Input: part model. Units: mm. Frame: model coordinates. A direction names the side the tool comes from. Coordinates: 2 decimals unless noted, no trailing zeros. Order: outer loops, then holes, each group sorted by start corner. A loop starts at its lowest first (then second) coordinate and runs counter-clockwise, first axis right, second up. Notation, with made-up numbers: M -8,49.25 L 17,49.25 A34 ccw 17,85.25 Z; hole C 67,75.25 d6. An arc over 180 degrees is marked long. Answer in a Markdown table with one row per item.
Autodesk Inventor part; units mm, degrees
ref_plane "Work Plane1" through (0, 10, 0) normal (0, 1, 0) x (-1, 0, 0)
ref_plane "YZ Plane" through (0, 0, 0) normal (1, 0, 0) x (0, 1, 0)
ref_plane "XY Plane" through (0, 0, 0) normal (0, 0, 1) x (1, 0, 0)
sketch "Sketch1" plane through (0, 0, 0) normal (0, 0, 1) x (1, 0, 0)
  line L0 (-50, 0) -> (0, 0)
  line L1 (0, 0) -> (50, 0)
  line L2 (-50, 0) -> (-50, 6)
  line L3 (-50, 6) -> (-33, 6)
  line L4 (-33, 6) -> (-33, 10)
  line L5 (-33, 10) -> (33, 10)
  line L6 (33, 10) -> (33, 6)
  line L7 (33, 6) -> (50, 6)
  line L8 (50, 6) -> (50, 0)
  point P0 (-33, 8)
  dimension "d0" = 100
  dimension "d1" = 12
  dimension "d2" = 20
  dimension "d3" = 17
  dimension "d4" = 83
revolve "Revolution1" add sketch "Sketch1" angle 360 about axis through (-50, 0, 0) along (1, 0, 0)
sketch "Sketch2" plane through (-50, 0, 0) normal (-1, 0, 0) x (0, 0, 1)
  circle A0 centre (0, 0) radius 6
hole "Hole1" at (-50, 0, 0) direction (1, 0, 0) diameter 5.1 depth 50 tip angle 118
ref_plane "Work Plane1" through (0, 10, 0) normal (0, 1, 0) x (-1, 0, 0)
sketch "Sketch3" plane through (0, 10, 0) normal (0, 1, 0) x (-1, 0, 0)
  line L0 (50, 6) -> (50, -6)
  point P0 (0, 0)
  point P1 (0, 0)
  dimension "d13" = 50
hole "Hole2" at (0, 10, 0) direction (0, -1, 0) diameter 5.1 depth 14 tip angle 118
chamfer "Chamfer1" distance 2 angle 45 2 edges at (-50, -6, 0) (50, -6, 0)
properties part number "05-spindel" material "Stainless Steel"
1) Material intervals for probe 1 along Z at (x, y) = (-19, 0); probe 2 along X at (y, z) = (0.5, 9); probe 3 along X at (y, z) = (3.75, 0), sorted ascending.
Resolved:
| item | result |
|---|---|
| probe 1 | z = -10 to -2.55, 2.55 to 10 |
| probe 2 | x = -33 to 33 |
| probe 3 | x = -50 to -2.55, 2.55 to 50 |
2) Cut plane D-D, the plane y = 7.75. Output: boundary loops of the cut face in (x, z).
Resolved:
| item | result |
|---|---|
| outline | M -33,-6.32 L 33,-6.32 L 33,6.32 L -33,6.32 Z; hole C 0,0 d5.1 |
3) Contact query for flat-ended pins moving along their axis: pin 1 (5 mm diameter, centred on x = -38.5, z = 5, fed in from -Y); pin 2 (10 mm diameter, centred on y = 7.5, z = -7, fed in from +X); pin 3 (5 mm diameter, centred on y = 8, z = -4.5, fed in from -X). Output: stop coordinate, or through.
Resolved:
| item | result |
|---|---|
| pin 1 | stops at y = -5.45 |
| pin 2 | stops at x = 48.74 |
| pin 3 | stops at x = -33 |
4) Cut plane C-C, the plane z = 8. Output: boundary loops of the cut face in (x, y), and give its area (3 significant figures).
Resolved:
| item | result |
|---|---|
| outline | M -33,-6 L 33,-6 L 33,6 L -33,6 Z |
| area | 792 mm2 |
5) Cut plane B-B, the plane x = -36.5. Output: boundary loops of the cut face in (y, z).
Resolved:
| item | result |
|---|---|
| outline | C 0,0 d12; hole C 0,0 d5.1 |
6) Mould query, pull axis Z, two halves, no side actions, for faces 4 (the face through (2.49, 2.9, -0.55)), 5 (the face through (0.46, -2.17, -9.76)), 6 (the face through (50, 0, 0)). Classes: +Z half, -Z half, draft (parallel to the pull), parting line (faces both ways), or undercut.
Resolved:
| item | result |
|---|---|
| face 4 | undercut |
| face 5 | parting line |
| face 6 | draft |
7) Cut plane A-A, the plane x = 41.5. Output: boundary loops of the cut face in (y, z), and give its area (3 significant figures).
Resolved:
| item | result |
|---|---|
| outline | C 0,0 d12 |
| area | 113 mm2 |
8) Reachability of faces 1 (the face through (33, 7, 0)), 2 (the face through (-40, -6, 0)), 3 (the face through (-50, 0, -3)) from +Z, -Z, +X, -X, +Y, -Y: full face, straight path, thin tool, end or side. Return the list, or none.
Resolved:
| item | result |
|---|---|
| face 1 | +X |
| face 2 | -X |
| face 3 | +Z, -Z, -X, +Y, -Y |
